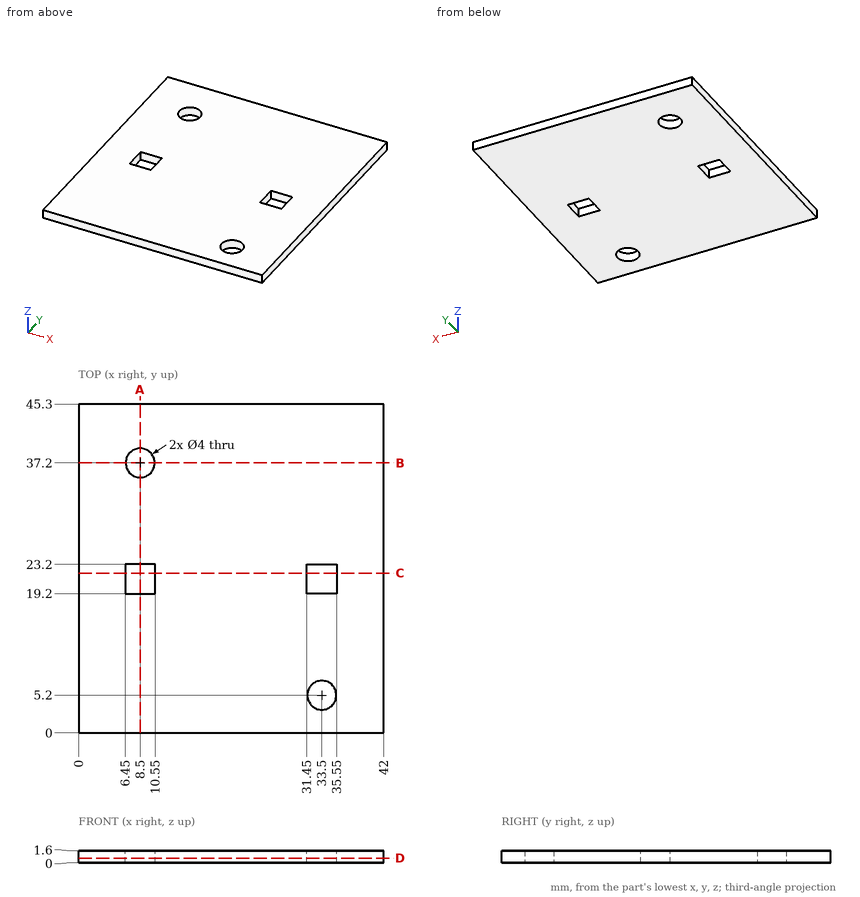
Geometry check sheet. Reference: drawing and pictorial views, mm from the part's lowest x, y, z. Round coordinates to 2 decimals unless told otherwise and drop trailing zeros. Write each loop counter-clockwise with the first axis right and the second up, starting at its lowest first coordinate (ties: lowest second). Pieces come first, ordered by that corner, then holes.
Item 1: Material ranges on line 1 along X through (y, z) = (23, 1.3); line 2 along Y through (x, z) = (33.5, 0.65); line 3 along Y through (x, z) = (8.5, 0.6), recorded low to high.
Determined:
line 1: x = 0 to 6.45, 10.55 to 31.45, 35.55 to 42
line 2: y = 0 to 3.2, 7.2 to 19.2, 23.2 to 45.3
line 3: y = 0 to 19.2, 23.2 to 35.2, 39.2 to 45.3
Item 2: Section check B-B (y = 37.2). Record the boundary of the cut face in (x, z).
Determined:
outline: (0, 0) - (6.5, 0) - (6.5, 1.6) - (0, 1.6) - close; (10.5, 0) - (42, 0) - (42, 1.6) - (10.5, 1.6) - close
Item 3: Section check A-A (x = 8.5). Record the boundary of the cut face in (y, z), plus the area to 3 significant figures.
Determined:
outline: (0, 0) - (19.2, 0) - (19.2, 1.6) - (0, 1.6) - close; (23.2, 0) - (35.2, 0) - (35.2, 1.6) - (23.2, 1.6) - close; (39.2, 0) - (45.3, 0) - (45.3, 1.6) - (39.2, 1.6) - close
area: 59.7 mm2
Item 4: Go/stop test with a flat-tipped pin: pin 1 Ø0.5 at (y, z) = (20.5, 0.5) entering from -X. Record where the tip stops, or that it passes through.
Determined:
pin 1: stops at x = 0
Item 5: Section check C-C (y = 22). Record the boundary of the cut face in (x, z), plus the area to 3 significant figures.
Determined:
outline: (0, 0) - (6.45, 0) - (6.45, 1.6) - (0, 1.6) - close; (10.55, 0) - (31.45, 0) - (31.45, 1.6) - (10.55, 1.6) - close; (35.55, 0) - (42, 0) - (42, 1.6) - (35.55, 1.6) - close
area: 54.1 mm2
Item 6: Section check D-D (z = 0.6). Record the boundary of the cut face in (x, y).
Determined:
outline: (0, 0) - (42, 0) - (42, 45.3) - (0, 45.3) - close; hole (6.45, 19.2) - (10.55, 19.2) - (10.55, 23.2) - (6.45, 23.2) - close; hole circle Ø4 at (8.5, 37.2); hole (31.45, 19.2) - (35.55, 19.2) - (35.55, 23.2) - (31.45, 23.2) - close; hole circle Ø4 at (33.5, 5.2)
